```python
from build123d import *

# Parameters (mm, degrees)
SKETCH1_R           = 18.5
BOSS_EXTRUDE1_DEPTH = 24.5
SKETCH2_R           = 18.1
BOSS_EXTRUDE2_DEPTH = 33.3
SKETCH4_R           = 6
BOSS_EXTRUDE3_DEPTH = 6
SKETCH5_R           = 3
BOSS_EXTRUDE4_DEPTH = 15
CUT_EXTRUDE1_DEPTH  = 12
FACE_DIAMENTIONS_R  = 1.5
CUT_EXTRUDE3_DEPTH  = 3


with BuildPart() as part:
    # Sketch1 → Boss-Extrude1 (new body)
    with BuildSketch(Plane.XY):
        Circle(SKETCH1_R)
    extrude(amount=BOSS_EXTRUDE1_DEPTH)

    # Sketch2 → Boss-Extrude2 (add)
    with BuildSketch(Plane.XY.offset(24.5)):
        Circle(SKETCH2_R)
    extrude(amount=BOSS_EXTRUDE2_DEPTH)

    # Sketch4 → Boss-Extrude3 (add)
    with BuildSketch(Plane(origin=(0, 0, 0), x_dir=(-1, 0, 0), z_dir=(0, 0, -1))):
        with Locations((0, 6.5)):
            Circle(SKETCH4_R)
    extrude(amount=BOSS_EXTRUDE3_DEPTH)

    # Sketch5 → Boss-Extrude4 (add)
    with BuildSketch(Plane(origin=(0, 0, -6), x_dir=(-1, 0, 0), z_dir=(0, 0, -1))):
        with Locations((0, 6.5)):
            Circle(SKETCH5_R)
    extrude(amount=BOSS_EXTRUDE4_DEPTH)

    # Sketch6 → Cut-Extrude1 (cut)
    with BuildSketch(Plane(origin=(0, 0, -21), x_dir=(-1, 0, 0), z_dir=(0, 0, -1))):
        with BuildLine():
            Line((2.75, 6.5), (2.75, 5.301042119))
            ThreePointArc((2.75, 5.301042119), (3, 6.5), (2.75, 7.698957881))
            Line((2.75, 7.698957881), (2.75, 6.5))
        make_face()
    extrude(amount=-CUT_EXTRUDE1_DEPTH, mode=Mode.SUBTRACT)

    # face diamentions → Cut-Extrude3 (cut)
    with BuildSketch(Plane(origin=(0, 0, 0), x_dir=(-1, 0, 0), z_dir=(0, 0, -1))):
        with Locations((-16, 0)):
            Circle(FACE_DIAMENTIONS_R)
        with Locations((8, 13.856406461)):
            Circle(FACE_DIAMENTIONS_R)
        with Locations((8, -13.856406461)):
            Circle(FACE_DIAMENTIONS_R)
        with Locations((16, 0)):
            Circle(FACE_DIAMENTIONS_R)
        with Locations((-8, -13.856406461)):
            Circle(FACE_DIAMENTIONS_R)
        with Locations((-8, 13.856406461)):
            Circle(FACE_DIAMENTIONS_R)
    extrude(amount=-CUT_EXTRUDE3_DEPTH, mode=Mode.SUBTRACT)


solid = part.part
```
Here's how the part is built. I have some questions about the finished solid (model axes, mm). A direction names the side the tool comes from. Round coordinates to 2 decimals unless told otherwise and drop trailing zeros. Order: outer loops, then holes, each group sorted by start corner. A loop starts at its lowest first (then second) coordinate and runs counter-clockwise, first axis right, second up. Notation, with made-up numbers: (24.5, 85) -> (82.5, 85) arc R11 ccw to (82.5, 101) -> close; hole circle Ø6 at (1.5, 30.5). An arc over 180 degrees is marked (long way). Use a Markdown table: item, result. Add a question column.
(1) Suppose I cut it at C-C, the plane z = 44. Please give me the cut outline in (x, y).
(2) Suppose I cut it at A-A, the plane y = -6. Please give me the cut outline in (x, z), and give its area (3 significant figures).
(3) For faces 4 (the face through (16, 0, 3)), 5 (the face through (13.6, -12.2, 24.5)), 6 (the face through (-2.75, 7, -15)), which set-ups out of +Z, -Z, +X, -X, +Y, -Y let a thin tool reach every point of the face, with its end or its side?
(4) For pin 1 Ø2.5 at (x, y) = (-8.5, 13.5) entering from -Z; pin 2 Ø8 at (y, z) = (9, 42) entering from +X; pin 3 Ø12 at (x, z) = (-3, 28.5) entering from +Y, each with a flat end and sliding along its axis, tell me the tip position at first contact or that it passes through.
(5) If we mould it in two halves opening along Y, with no side actions, what happens to faces 1 (the face through (-4.01, -18.06, 12.08)), 2 (the face through (17.5, 0.07, 1.48)), 3 (the face through (0, 0, 57.8))? For each: released by +Y, released by -Y, zero draft, split by the parting line, or undercut.
(6) I need wall thicknesses on line 1 along Y through (x, z) = (-8, 2); line 2 along Z through (x, y) = (-11, 1.5); line 3 along X through (y, z) = (-6, 3.5). Which ranges of each line are inside material? Lowest first, please.
(7) Suppose I cut it at D-D, the plane y = -11. Please give me the cut outline in (x, z), and give its area (3 significant figures).
(8) Suppose I cut it at B-B, the plane x = 0. Please give me the cut outline in (y, z).
Verdict:
| question | item | result |
|---|---|---|
| 1 | outline | circle Ø36.2 at (0, 0) |
| 2 | outline | (-17.5, 0) -> (17.5, 0) -> (17.5, 24.5) -> (17.08, 24.5) -> (17.08, 57.8) -> (-17.08, 57.8) -> (-17.08, 24.5) -> (-17.5, 24.5) -> close |
| 2 | area | 1,990 mm2 |
| 3 | face 4 | -Z |
| 3 | face 5 | +Z |
| 3 | face 6 | -Z, -X, +Y, -Y |
| 4 | pin 1 | z = 0 |
| 4 | pin 2 | x = 17.4 |
| 4 | pin 3 | y = 18.5 |
| 5 | face 1 | split by the parting line |
| 5 | face 2 | undercut |
| 5 | face 3 | zero draft |
| 6 | line 1 | -16.68 to -15.36, -12.36 to 12.36, 15.36 to 16.68 |
| 6 | line 2 | 0 to 57.8 |
| 6 | line 3 | -17.5 to 17.5 |
| 7 | outline | (-14.87, 0) -> (14.87, 0) -> (14.87, 24.5) -> (14.37, 24.5) -> (14.37, 57.8) -> (-14.37, 57.8) -> (-14.37, 24.5) -> (-14.87, 24.5) -> close |
| 7 | area | 1,690 mm2 |
| 8 | outline | (-18.5, 0) -> (0.5, 0) -> (0.5, -6) -> (3.5, -6) -> (3.5, -21) -> (9.5, -21) -> (9.5, -6) -> (12.5, -6) -> (12.5, 0) -> (18.5, 0) -> (18.5, 24.5) -> (18.1, 24.5) -> (18.1, 57.8) -> (-18.1, 57.8) -> (-18.1, 24.5) -> (-18.5, 24.5) -> close |
